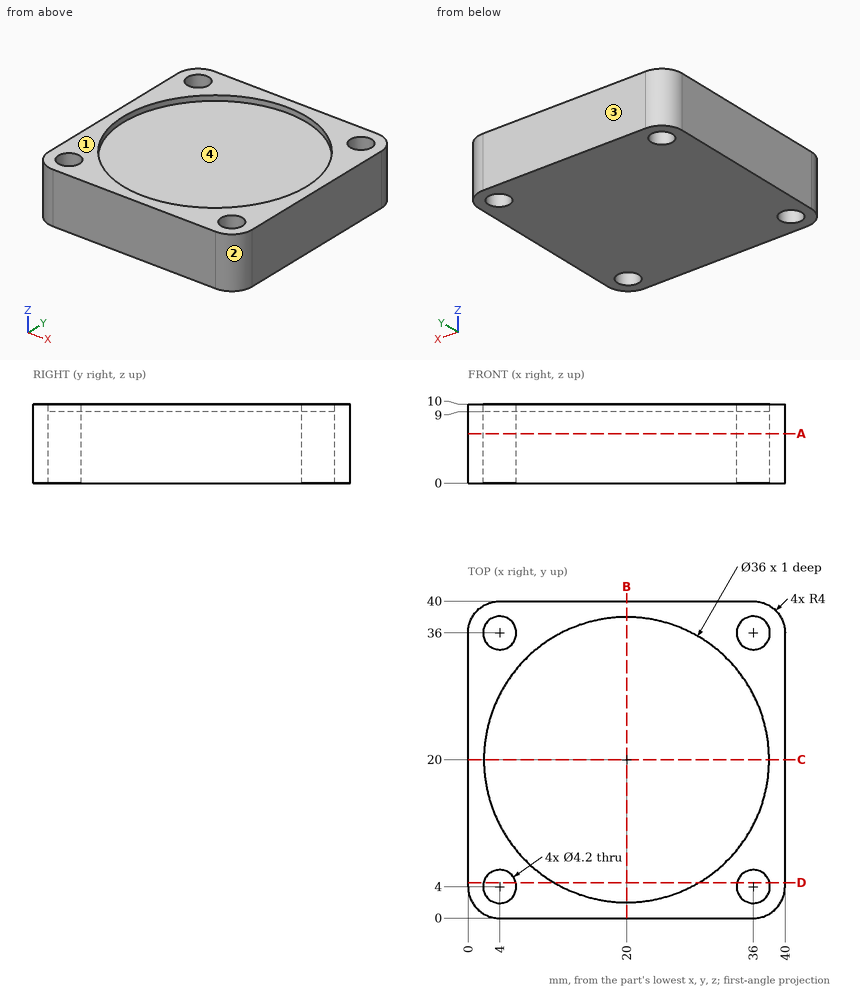
Verification items for this drawing (mm, ordinates from the low corner). Give positions to 0.01 mm unless a question says otherwise; leave off trailing zeros. Loops run counter-clockwise (first coordinate to the right, second up) from the corner with the lowest first, then second, coordinate; pieces in that order, holes last.
(1) Section check D-D on y = 4.5. Record the cut outline in (x, z), then the cut area to 3 significant figures.
From the geometry:
outline: (0, 0) - (1.96, 0) - (1.96, 10) - (0, 10) - close; (6.04, 0) - (33.96, 0) - (33.96, 10) - (29.15, 10) - (29.15, 9) - (10.85, 9) - (10.85, 10) - (6.04, 10) - close; (38.04, 0) - (40, 0) - (40, 10) - (38.04, 10) - close
area: 300 mm2
(2) Release check for a two-part mould opening along Y. For the marked faces 1, 2, 3 and 4 record: released by +Y, released by -Y, zero draft, split by the parting line, or undercut.
From the geometry:
face 1: zero draft
face 2: released by -Y
face 3: released by +Y
face 4: undercut
(3) Depth check by flat-ended pin: pin 1 Ø4 at (x, y) = (8.5, 16) entering from +Z. Enter the tip coordinate at first touch or a pass-through.
From the geometry:
pin 1: stops at z = 9
(4) Section check A-A on z = 6.25. Record the cut outline in (x, y), then the cut area to 3 significant figures.
From the geometry:
outline: (0, 4) arc R4 ccw to (4, 0) - (36, 0) arc R4 ccw to (40, 4) - (40, 36) arc R4 ccw to (36, 40) - (4, 40) arc R4 ccw to (0, 36) - close; hole circle Ø4.2 at (4, 4); hole circle Ø4.2 at (4, 36); hole circle Ø4.2 at (36, 4); hole circle Ø4.2 at (36, 36)
area: 1,530 mm2
(5) Section check B-B on x = 20. Record the cut outline in (y, z).
From the geometry:
outline: (0, 0) - (40, 0) - (40, 10) - (38, 10) - (38, 9) - (2, 9) - (2, 10) - (0, 10) - close
(6) Thickness scan on L1, parallel to Y at x = 4, z = 3.5; L2, parallel to Y at x = 20, z = 9.75. Record the ranges inside material, lowest first.
From the geometry:
L1: y = 0 to 1.9, 6.1 to 33.9, 38.1 to 40
L2: y = 0 to 2, 38 to 40
